```python
from build123d import *

# Parameters (mm, degrees)
SKETCH1_W           = 22.5
SKETCH1_H           = 25
SKETCH1_R           = 7.5
BOSS_EXTRUDE1_DEPTH = 24
CUT_EXTRUDE4_DEPTH  = 30.807717122
SKETCH7_W           = 10
SKETCH7_H           = 25
BOSS_EXTRUDE2_DEPTH = 24
SKETCH8_R           = 4.1
CUT_EXTRUDE5_DEPTH  = 48


with BuildPart() as part:
    # Sketch1 → Boss-Extrude1 (new body)
    with BuildSketch(Plane(origin=(0, 0, 0), x_dir=(1, 0, 0), z_dir=(0, 1, 0))):
        with Locations((1.25, 0)):
            Rectangle(SKETCH1_W, SKETCH1_H)
        with Locations(Location((0, 0, 0), (0, 0, 270))):
            Circle(SKETCH1_R, mode=Mode.SUBTRACT)
    extrude(amount=BOSS_EXTRUDE1_DEPTH)

    # Sketch5 → Cut-Extrude4 (cut, through all)
    with BuildSketch(Plane.XZ):
        Polygon((12.5, 12.5), (6.5, 12.5), (6.5, 4.363484846), (6.1, 4.363484846), (6.1, -4.363484846), (6.5, -4.363484846), (6.5, -12.5), (12.5, -12.5), align=None)
    extrude(amount=-CUT_EXTRUDE4_DEPTH, mode=Mode.SUBTRACT)

    # Sketch7 → Boss-Extrude2 (add)
    with BuildSketch(Plane.XZ):
        with Locations((-15, 0)):
            Rectangle(SKETCH7_W, SKETCH7_H)
    extrude(amount=-BOSS_EXTRUDE2_DEPTH)

    # Sketch8 → Cut-Extrude5 (cut)
    with BuildSketch(Plane.XY.offset(12.5)):
        with Locations((-14, 12)):
            Circle(SKETCH8_R)
    extrude(amount=-CUT_EXTRUDE5_DEPTH, mode=Mode.SUBTRACT)


solid = part.part
```
Design review of the part built by this model. Coordinates are the model's own, in mm. Coordinates: 2 decimals unless noted, no trailing zeros. Loops run counter-clockwise (first coordinate to the right, second up) from the corner with the lowest first, then second, coordinate; pieces in that order, holes last. Notation, with made-up numbers: (-20.75, 70) - (4.25, 70) arc R19 cw to (4.25, 89) - close; hole circle Ø10 at (46.5, 73.5). An arc over 180 degrees is marked (long way). Use CSV: the item, a comma, the result in double quotes. Start each with the question number.
1) Consider section C-C on y = 12. Write out the cut boundary in (x, z), then the cut area to 3 significant figures.
2) Consider section D-D on z = 5.25. Write out the cut boundary in (x, y), then the cut area to 3 significant figures.
3) Wall thickness on L1, parallel to Y at x = -14, z = 2; L2, parallel to X at y = 13, z = 5; L3, parallel to Z at x = 0, y = 9.5: over which ranges is each line inside the solid? List them lowest first. Write a range as from..to.
4) Consider section A-A on x = 0. Write out the cut boundary in (y, z).
5) Consider section B-B on z = -10.25. Write out the cut boundary in (x, y).
6) The part is to be moulded in two halves that separate along X. For faces 1 (the flat face through (6.5, 12, 8)), 2 (the cylindrical face through (-7.495, 11.832, -0.265)), 3 (the flat face through (-10, 0, 0)), say which applies: +X half, -X half, draft (parallel to the pull), parting line (faces both ways), or undercut.
Geometry says:
1,outline,"(-20, -12.5) - (-18.1, -12.5) - (-18.1, 12.5) - (-20, 12.5) - close; (-9.9, -12.5) - (6.5, -12.5) - (6.5, -4.36) - (6.1, -4.36) arc R7.5 cw (long way) to (6.1, 4.36) - (6.5, 4.36) - (6.5, 12.5) - (-9.9, 12.5) - close"
1,area,"286 mm^2"
2,outline,"(-20, 0) - (-5.36, 0) - (-5.36, 24) - (-20, 24) - close; (5.36, 0) - (6.5, 0) - (6.5, 24) - (5.36, 24) - close; hole circle Ø8.2 at (-14, 12)"
2,area,"326 mm^2"
3,L1,"0..7.9, 16.1..24"
3,L2,"-20..-17.98, -10.02..-5.59, 5.59..6.5"
3,L3,"-12.5..-7.5, 7.5..12.5"
4,outline,"(0, -12.5) - (24, -12.5) - (24, -7.5) - (0, -7.5) - close; (0, 7.5) - (24, 7.5) - (24, 12.5) - (0, 12.5) - close"
5,outline,"(-20, 0) - (6.5, 0) - (6.5, 24) - (-20, 24) - close; hole circle Ø8.2 at (-14, 12)"
6,face 1,"+X half"
6,face 2,"undercut"
6,face 3,"draft"
